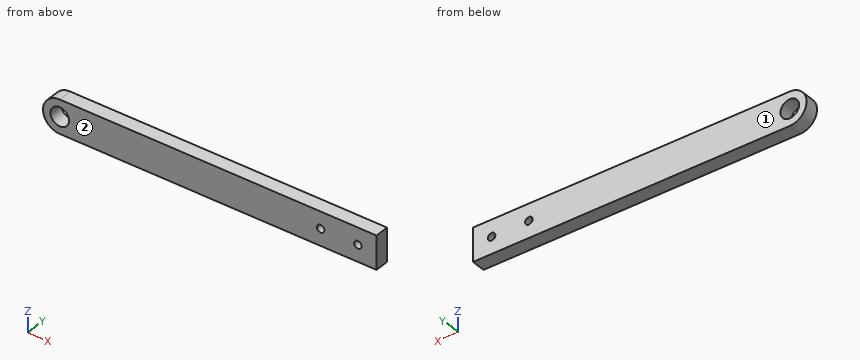
```python
from build123d import *

# Parameters (mm, degrees)
BOSS_EXTRUDE1_DEPTH = 7.5
SKETCH2_R           = 5
SKETCH2_R_2         = 2
CUT_EXTRUDE1_DEPTH  = 171.403198327


with BuildPart() as part:
    # Sketch1 → Boss-Extrude1 (new body)
    with BuildSketch(Plane(origin=(0, 0, 0), x_dir=(1, 0, 0), z_dir=(0, 1, 0))):
        with BuildLine():
            Line((0, 9), (170, 9))
            Line((170, 9), (170, -9))
            Line((170, -9), (0, -9))
            ThreePointArc((0, -9), (-9, 0), (0, 9))
        make_face()
    extrude(amount=BOSS_EXTRUDE1_DEPTH)

    # Sketch2 → Cut-Extrude1 (cut, through all)
    with BuildSketch(Plane(origin=(0, 7.5, 0), x_dir=(1, 0, 0), z_dir=(0, 1, 0))):
        with Locations(Location((0, 0, 0), (0, 0, 270))):
            Circle(SKETCH2_R)
        with Locations(Location((160, 0, 0), (0, 0, 270))):
            Circle(SKETCH2_R_2)
        with Locations(Location((140, 0, 0), (0, 0, 270))):
            Circle(SKETCH2_R_2)
    extrude(amount=-CUT_EXTRUDE1_DEPTH, mode=Mode.SUBTRACT)


solid = part.part
```
Work out the finished part from the listing and answer in its coordinate system (mm). Face numbers are marked on the shaded views. Coordinates: 2 decimals unless noted, no trailing zeros. Order: outer loops, then holes, each group sorted by start corner. A loop starts at its lowest first (then second) coordinate and runs counter-clockwise, first axis right, second up. Notation, with made-up numbers: M 87.25,29 L 94.25,29 A22 cw 94.25,53 Z; hole C 85.25,-18 d7. An arc over 180 degrees is marked long. Use CSV: the item, a comma, the result in double quotes.
1) Section A-A on z = 0 is taken. Write down the section's boundary in (x, y), plus the area to 3 significant figures.
Worked out:
outline,"M -9,0 L -5,0 L -5,7.5 L -9,7.5 Z; M 5,0 L 138,0 L 138,7.5 L 5,7.5 Z; M 142,0 L 158,0 L 158,7.5 L 142,7.5 Z; M 162,0 L 170,0 L 170,7.5 L 162,7.5 Z"
area,"1,210 mm^2"
2) Consider line 1 (X direction, y = 3, z = 0); line 2 (X direction, y = 3.25, z = -0.5); line 3 (Z direction, x = 160, y = 2). Determine where each line is inside the solid, lowest interval first. Write a range as [from, to].
Worked out:
line 1,"x = [-9, -5], [5, 138], [142, 158], [162, 170]"
line 2,"x = [-8.99, -4.97], [4.97, 138.06], [141.94, 158.06], [161.94, 170]"
line 3,"z = [-9, -2], [2, 9]"
3) Section C-C on x = 140 is taken. Write down the section's boundary in (y, z).
Worked out:
outline,"M 0,-9 L 7.5,-9 L 7.5,-2 L 0,-2 Z; M 0,2 L 7.5,2 L 7.5,9 L 0,9 Z"
4) Determine the mould class of the marked faces 1 and 2 for opening direction Y: released by +Y, released by -Y, zero draft, split by the parting line, or undercut.
Worked out:
face 1,"released by +Y"
face 2,"released by -Y"
5) Section B-B on y = 6 is taken. Write down the section's boundary in (x, z), plus the area to 3 significant figures.
Worked out:
outline,"M 0,-9 L 170,-9 L 170,9 L 0,9 A9 ccw Z; hole C 0,0 d10; hole C 140,0 d4; hole C 160,0 d4"
area,"3,080 mm^2"
6) Section D-D on z = 7.5 is taken. Write down the section's boundary in (x, y).
Worked out:
outline,"M -4.97,0 L 170,0 L 170,7.5 L -4.97,7.5 Z"
